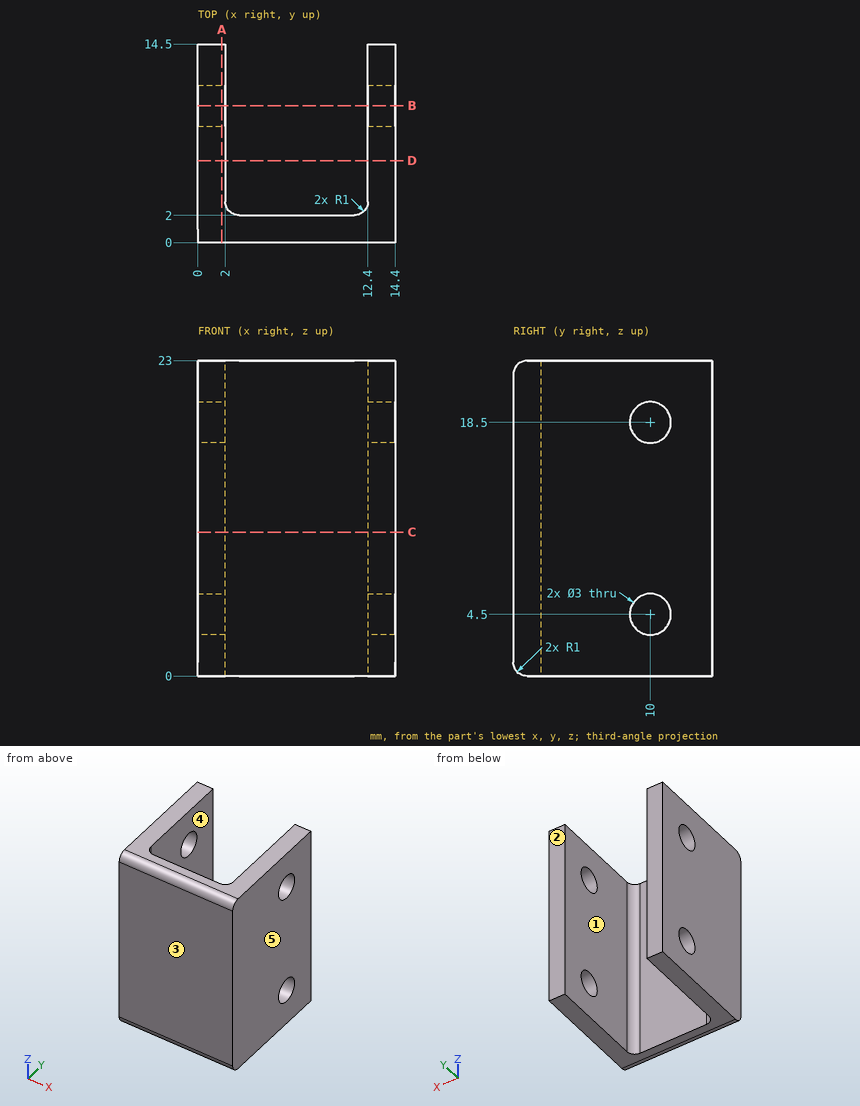
Check sheet for the drawn part. Datum: minimum x, y, z corner. Units: mm. A direction names the side the tool comes from. Give positions to 0.01 mm unless a question says otherwise; leave off trailing zeros. Loops run counter-clockwise (first coordinate to the right, second up) from the corner with the lowest first, then second, coordinate; pieces in that order, holes last. Notation, with made-up numbers: (-11, 55) - (-3, 55) arc R27 ccw to (-3, 94) - close; hole circle Ø3 at (36, -16.5). An arc over 180 degrees is marked (long way). Write each question's results on one line, items separated by ' | '.
1) Mould release check, pull along X, two halves, no side actions. Record for the marked faces 3, 4 and 5: pulls with the +X half, pulls with the -X half, needs draft (parallel to the pull), parting line crosses it, or undercut.
Solution:
face 3: needs draft | face 4: undercut | face 5: pulls with the +X half
2) Tool access check on the marked faces 1 and 2. Record the directions out of +Z, -Z, +X, -X, +Y, -Y that give a thin tool (end or side, any length) a straight path to the whole face; none if there is none.
Solution:
face 1: +Z, -Z, +Y | face 2: +Z, -Z, +X, -X, +Y
3) Sectioned sample at B-B on y = 10. Record the boundary of the cut face in (x, z).
Solution:
outline: (0, 0) - (2, 0) - (2, 3) - (0, 3) - close; (0, 6) - (2, 6) - (2, 17) - (0, 17) - close; (0, 20) - (2, 20) - (2, 23) - (0, 23) - close; (12.4, 0) - (14.4, 0) - (14.4, 3) - (12.4, 3) - close; (12.4, 6) - (14.4, 6) - (14.4, 17) - (12.4, 17) - close; (12.4, 20) - (14.4, 20) - (14.4, 23) - (12.4, 23) - close
4) Sectioned sample at C-C on z = 10.5. Record the boundary of the cut face in (x, y), plus the area to 3 significant figures.
Solution:
outline: (0, 0) - (14.4, 0) - (14.4, 14.5) - (12.4, 14.5) - (12.4, 3) arc R1 cw to (11.4, 2) - (3, 2) arc R1 cw to (2, 3) - (2, 14.5) - (0, 14.5) - close | area: 79.2 mm2
5) Sectioned sample at D-D on y = 6. Record the boundary of the cut face in (x, z).
Solution:
outline: (0, 0) - (2, 0) - (2, 23) - (0, 23) - close; (12.4, 0) - (14.4, 0) - (14.4, 23) - (12.4, 23) - close
6) Depth check by flat-ended pin: P1, Ø1.8, axis at y = 10, z = 18.5, coming from the +X side; P2, Ø1.5, axis at x = 4, z = 9.5, coming from the +Y side. Enter the tip coordinate at first touch or a pass-through.
Solution:
P1: through | P2: y = 2
7) Material ranges on L1, parallel to Y at x = 13.65, z = 18.5; L2, parallel to X at y = 7, z = 22; L3, parallel to Y at x = 3.75, z = 16.5, recorded low to high. Write a range as from..to.
Solution:
L1: 0..8.5, 11.5..14.5 | L2: 0..2, 12.4..14.4 | L3: 0..2
8) Sectioned sample at A-A on x = 1.75. Record the boundary of the cut face in (y, z).
Solution:
outline: (0, 1) arc R1 ccw to (1, 0) - (14.5, 0) - (14.5, 23) - (1, 23) arc R1 ccw to (0, 22) - close; hole circle Ø3 at (10, 4.5); hole circle Ø3 at (10, 18.5)
